Geometry check sheet. Reference: the model listing, model coordinates, mm. Coordinates: 2 decimals unless noted, no trailing zeros. Loops run counter-clockwise (first coordinate to the right, second up) from the corner with the lowest first, then second, coordinate; pieces in that order, holes last. Notation, with made-up numbers: (40, 88.5) - (97, 88.5) arc R12 cw to (97, 97.5) - close; hole circle Ø7 at (-27, -4). An arc over 180 degrees is marked (long way). Write each question's results on one line, items separated by ' | '. Start each with the question number.
(1) Sectioned sample at A-A (x = 18.5). Enter the section's corners in (y, z), plus the area to 3 significant figures.
(2) Go/stop test with flat-tipped pins: pin 1 Ø1.5 at (y, z) = (-2.5, 1.5) entering from +X; pin 2 Ø1.9 at (x, z) = (13.5, 0.5) entering from -Y; pin 3 Ø0.7 at (y, z) = (2.5, 0) entering from -X; pin 4 Ø0.5 at (x, z) = (19.5, 1) entering from +Y. Record where each tip stops, or that it passes through.
(3) Sectioned sample at B-B (x = 46). Enter the section's corners in (y, z).
(4) Material ranges on probe 1 along X at (y, z) = (1, 0.05); probe 2 along Y at (x, z) = (7.5, 1.4); probe 3 along Y at (x, z) = (54, -1.15), recorded low to high.
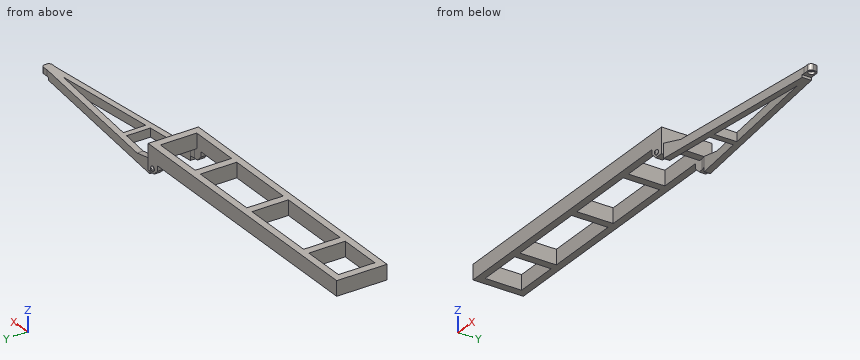
from build123d import *

# Parameters (mm, degrees)
F1_DEPTH  = 1.72
F3_DEPTH  = 0.8
F5_DEPTH  = 2
F7_DEPTH  = 2.901
F8_R      = 0.2889302174
F9_DEPTH  = 0.2
F10_SIZE  = 0.15
F12_W     = 1.3
F12_H     = 0.3
F13_DEPTH = 6.001
F14_R     = 0.4
F15_R     = 0.35
F16_DEPTH = 0.3


with BuildPart() as f1:
    # F0 (on Top) → F1 (new body)
    with BuildSketch(Plane.XY):
        Polygon((0.9, 0), (0, 0), (0, -2.9), (32.5, -2.9), (32.5, 0), (31.6, 0), (31.6, -2.1), (25.6, -2.1), (25.6, 0), (24.7, 0), (24.7, -2.1), (16.7, -2.1), (16.7, 0), (15.8, 0), (15.8, -2.1), (6.9, -2.1), (6.9, 0), (6, 0), (6, -2.1), (0.9, -2.1), align=None)
    extrude(amount=F1_DEPTH)

    # F2 (on face) → F3 (join, through all)
    with BuildSketch(Plane.XZ.offset(2.9)):
        Polygon((30.9, 0), (30.9, -0.6), (32, -1.7), (32.5, -1.7), (32.5, 0), align=None)
    extrude(amount=-F3_DEPTH)

    # F4 (on face) → F5 (join)
    with BuildSketch(Plane(origin=(0, 0, -1.7), x_dir=(1, 0, 0), z_dir=(0, 0, -1))):
        Polygon((53.5, 0.5), (32.5, 2.7), (32.5, 2.1), (32, 2.1), (32.5, 1.9961692123), (38.5, 1.3675977837), (38.5, 0), (39.2, 0), (39.2, 1.2942644504), (51.5543424806, 0), (54.5, 0), (54.5, 0.5), align=None)
    extrude(amount=-F5_DEPTH)

    # F6 (on face) → F7 (cut, through all)
    with BuildSketch(Plane.XZ.offset(2.9)):
        Polygon((54.5, 0.3), (32.5, 0.3), (32.5, 0), (35.1124355653, -0.7), (54.5, -0.7), align=None)
        Polygon((32.5, -1.6719941439), (32.5, -1.2), (31.5, -1.2), (32, -1.7), (32.5, -1.7), (32.6045192778, -1.7), align=None)
    extrude(amount=-F7_DEPTH, mode=Mode.SUBTRACT)

    # F8 (on face) → F9 (join)
    with BuildSketch(Plane.XZ.offset(2.9)):
        with Locations((31.7, -0.7)):
            Circle(F8_R)
    extrude(amount=F9_DEPTH)

    # F10
    f10_edges = [f1.edges().sort_by_distance(p)[0] for p in [
        (31.41107, -3.1, -0.7),
    ]]
    chamfer(f10_edges, length=F10_SIZE)

    # F11: F1 across face


with BuildPart() as f1_1:
    add(f1.part)
    add(f1.part.mirror(Plane(origin=(16.25, 0, 0.86), x_dir=(-1, 0, 0), z_dir=(0, 1, 0))))

    # F12 (on face) → F13 (cut, through all)
    with BuildSketch(Plane(origin=(0, 2.9, 0), x_dir=(-1, 0, 0), z_dir=(0, 1, 0))):
        with Locations((-53.85, -1.55)):
            Rectangle(F12_W, F12_H)
    extrude(amount=-F13_DEPTH, mode=Mode.SUBTRACT)

    # F14
    f14_edges = [f1_1.edges().sort_by_distance(p)[0] for p in [
        (54.5, 0.5, -1.05),
        (54.5, -0.5, -1.05),
    ]]
    fillet(f14_edges, radius=F14_R)

    # F15 (on face) → F16 (cut)
    with BuildSketch(Plane(origin=(0, 0, -1.4), x_dir=(1, 0, 0), z_dir=(0, 0, -1))):
        with Locations((54, 0)):
            Circle(F15_R)
    extrude(amount=-F16_DEPTH, mode=Mode.SUBTRACT)


solid = f1_1.part
Outcome:
1) outline: (-2.9, 0) - (-2.1, 0) - (-2.1, 1.72) - (-2.9, 1.72) - close; (2.1, 0) - (2.9, 0) - (2.9, 1.72) - (2.1, 1.72) - close | area: 2.75 mm2
2) pin 1: stops at x = 32.5 | pin 2: stops at y = -2.9 | pin 3: stops at x = 0 | pin 4: stops at y = 2.9
3) outline: (-1.29, -1.7) - (-0.58, -1.7) - (-0.58, -0.7) - (-1.29, -0.7) - close; (0.58, -1.7) - (1.29, -1.7) - (1.29, -0.7) - (0.58, -0.7) - close
4) probe 1: x = 0 to 0.9, 6 to 6.9, 15.8 to 16.7, 24.7 to 25.6, 31.6 to 32.5 | probe 2: y = -2.9 to -2.1, 2.1 to 2.9 | probe 3: y = -0.5 to -0.35, 0.35 to 0.5
